The listing builds one solid part. Answer for the finished solid, in the listing's coordinates (mm). Round coordinates to 2 decimals unless told otherwise and drop trailing zeros. Loops run counter-clockwise (first coordinate to the right, second up) from the corner with the lowest first, then second, coordinate; pieces in that order, holes last. Notation, with made-up numbers: (9, 11) -> (14, 11) arc R19 ccw to (14, 37) -> close; hole circle Ø4 at (-17, 5.5). An arc over 180 degrees is marked (long way). Write each question's results on one line, items separated by ' | '. Start each with the question number.
from build123d import *

# Parameters (mm, degrees)
SKETCH1_W                                     = 99.2004
SKETCH1_H                                     = 46
BOSS_EXTRUDE1_DEPTH                           = 1.6002
CSK_FOR_0_FLAT_HEAD_SOCKET_CAP_SCREW1_A_COUNT = 2
CSK_FOR_0_FLAT_HEAD_SOCKET_CAP_SCREW1_A_PITCH = 41
CSK_FOR_0_FLAT_HEAD_SOCKET_CAP_SCRE_2_COUNT   = 2
CSK_FOR_0_FLAT_HEAD_SOCKET_CAP_SCRE_2_PITCH   = 96.358236597
CSK_FOR_0_FLAT_HEAD_SOCKET_CAP_SCRE_3_COUNT   = 2
CSK_FOR_0_FLAT_HEAD_SOCKET_CAP_SCRE_3_PITCH   = 87.2004


with BuildPart() as part:
    # Sketch1 → Boss-Extrude1 (new body)
    with BuildSketch(Plane(origin=(0, 0, 0), x_dir=(0, 0, -1), z_dir=(1, 0, 0))):
        with Locations((49.6002, 23)):
            Rectangle(SKETCH1_W, SKETCH1_H)
    extrude(amount=BOSS_EXTRUDE1_DEPTH)

    # Sketch4 → CSK for #0 Flat Head Socket Cap Screw1 (revolve, cut)
    with BuildSketch(Plane(origin=(1.6002, 43.5, -6), x_dir=(0, 0, -1), z_dir=(0, 1, 0))):
        Polygon((0, 0), (0, 1.6002), (0.889, 1.6002), (0.889, 0.993458156), (1.7526, 0), align=None)
    csk_for_0_flat_head_socket_cap_screw1 = revolve(axis=Axis((7.9502, 43.5, -6), (-1, 0, 0)), mode=Mode.SUBTRACT)

    # CSK for #0 Flat Head Socket Cap Screw1 a: CSK for #0 Flat Head Socket Cap Screw1 ×2
    with Locations(*[(0, -i * CSK_FOR_0_FLAT_HEAD_SOCKET_CAP_SCREW1_A_PITCH, 0) for i in range(1, CSK_FOR_0_FLAT_HEAD_SOCKET_CAP_SCREW1_A_COUNT)]):
        add(csk_for_0_flat_head_socket_cap_screw1, mode=Mode.SUBTRACT)

    # CSK for _0 Flat Head Socket Cap Scre 2: CSK for #0 Flat Head Socket Cap Screw1 ×2
    with Locations(*[Vector(0, -0.425495541, -0.904960521) * (i * CSK_FOR_0_FLAT_HEAD_SOCKET_CAP_SCRE_2_PITCH) for i in range(1, CSK_FOR_0_FLAT_HEAD_SOCKET_CAP_SCRE_2_COUNT)]):
        add(csk_for_0_flat_head_socket_cap_screw1, mode=Mode.SUBTRACT)

    # CSK for _0 Flat Head Socket Cap Scre 3: CSK for #0 Flat Head Socket Cap Screw1 ×2
    with Locations(*[(0, 0, -i * CSK_FOR_0_FLAT_HEAD_SOCKET_CAP_SCRE_3_PITCH) for i in range(1, CSK_FOR_0_FLAT_HEAD_SOCKET_CAP_SCRE_3_COUNT)]):
        add(csk_for_0_flat_head_socket_cap_screw1, mode=Mode.SUBTRACT)


solid = part.part
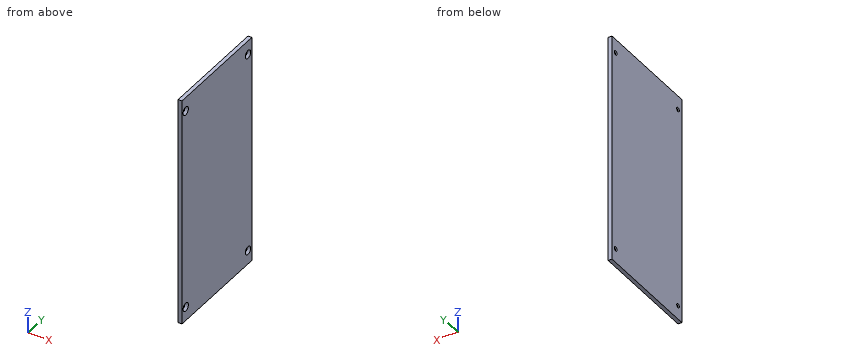
Item 1: Each of these flat-tipped pins is pushed along its axis until it touches: pin 1 Ø1.1 at (y, z) = (2.5, -6) entering from +X (3 decimals); pin 2 Ø2 at (y, z) = (43.5, -93.2) entering from +X. Where does it stop, or does it pass through?
Item 2: Straight lines are drawn through the part: L1, parallel to Y at x = 0.25, z = -6; L2, parallel to Z at x = 0.55, y = 2.5; L3, parallel to Z at x = 0.9, y = 42.5. For each, find the intervals that lie inside material, in ascending order. Write a range as [from, to].
Item 3: The part is cut by section B-B, the plane z = -6. Give the vertices of the cut face in (x, y).
Item 4: The part is cut by section A-A, the plane y = 43.5. Give the vertices of the cut face in (x, z), plus the area to 3 significant figures.
Report:
1) pin 1: passes through | pin 2: stops at x = 0.73
2) L1: y = [0, 1.61], [3.39, 42.61], [44.39, 46] | L2: z = [-99.2, -94.09], [-92.31, -6.89], [-5.11, 0] | L3: z = [-99.2, -93.76], [-92.64, -6.56], [-5.44, 0]
3) outline: (0, 0) -> (1.6, 0) -> (1.6, 0.75) -> (0.61, 1.61) -> (0, 1.61) -> close; (0, 3.39) -> (0.61, 3.39) -> (1.6, 4.25) -> (1.6, 41.75) -> (0.61, 42.61) -> (0, 42.61) -> close; (0, 44.39) -> (0.61, 44.39) -> (1.6, 45.25) -> (1.6, 46) -> (0, 46) -> close
4) outline: (0, -99.2) -> (1.6, -99.2) -> (1.6, -94.95) -> (0.61, -94.09) -> (0, -94.09) -> close; (0, -92.31) -> (0.61, -92.31) -> (1.6, -91.45) -> (1.6, -7.75) -> (0.61, -6.89) -> (0, -6.89) -> close; (0, -5.11) -> (0.61, -5.11) -> (1.6, -4.25) -> (1.6, 0) -> (0, 0) -> close | area: 151 mm2
